```python
from build123d import *

# Parameters (mm, degrees)
SKETCH1_R           = 2.1
BOSS_EXTRUDE1_DEPTH = 1.6
SKETCH3_W           = 0.5
SKETCH3_H           = 0.75
SKETCH3_W_2         = 0.75
SKETCH3_H_2         = 0.5
CUT_EXTRUDE1_DEPTH  = 0.5
SKETCH4_R           = 1.25
BOSS_EXTRUDE2_DEPTH = 7.5


with BuildPart() as part:
    # Sketch1 → Boss-Extrude1 (new body)
    with BuildSketch(Plane.XY):
        Circle(SKETCH1_R)
    extrude(amount=BOSS_EXTRUDE1_DEPTH)

    # Sketch2 → Cut-Revolve1 (revolve, cut)
    with BuildSketch(Plane(origin=(0, 0, 0), x_dir=(1, 0, 0), z_dir=(0, 1, 0))):
        with BuildLine():
            Line((-2.1, -0.8), (-2.1, 0))
            Line((-2.1, 0), (-1.3, 0))
            ThreePointArc((-1.3, 0), (-1.865685425, -0.234314575), (-2.1, -0.8))
        make_face()
    revolve(axis=Axis((0, 0, 0), (0, 0, 1)), mode=Mode.SUBTRACT)

    # Sketch3 → Cut-Extrude1 (cut)
    with BuildSketch(Plane(origin=(0, 0, 0), x_dir=(-1, 0, 0), z_dir=(0, 0, -1))):
        with Locations((0, -0.625)):
            Rectangle(SKETCH3_W, SKETCH3_H)
        with Locations((0.625, 0)):
            Rectangle(SKETCH3_W_2, SKETCH3_H_2)
        with Locations((-0.625, 0)):
            Rectangle(SKETCH3_W_2, SKETCH3_H_2)
        with Locations((0, 0.625)):
            Rectangle(SKETCH3_W, SKETCH3_H)
        Rectangle(SKETCH3_W, SKETCH3_H_2)
    extrude(amount=-CUT_EXTRUDE1_DEPTH, mode=Mode.SUBTRACT)

    # Sketch4 → Boss-Extrude2 (add)
    with BuildSketch(Plane.XY.offset(1.6)):
        Circle(SKETCH4_R)
    extrude(amount=BOSS_EXTRUDE2_DEPTH)


solid = part.part
```
Part model, mm, in its own coordinate system. A direction names the side the tool comes from. Coordinates: 2 decimals unless noted, no trailing zeros. Order: outer loops, then holes, each group sorted by start corner. A loop starts at its lowest first (then second) coordinate and runs counter-clockwise, first axis right, second up. Notation, with made-up numbers: (39, 10) - (77, 10) arc R25 cw to (77, 39) - close; hole circle Ø1 at (52.5, 89). An arc over 180 degrees is marked (long way). Return JSON: item names as keys, results as strings. Group by question number.
Item 1: Which spindle directions (+Z, -Z, +X, -X, +Y, -Y) get a long thin tool onto all of the face, cutting with end or side? Do faces 1 (the face through (1, -1, 1.6)), 2 (the face through (2.003, 0.631, 1.194)). Say none if no direction does.
Item 2: Drill centre lines: probe 1 along X at (y, z) = (0.05, 2.25); probe 2 along Z at (x, y) = (-1, 0.9); probe 3 along Z at (x, y) = (0, -0.7). Where is each one in solid material? Low to high. Write a range as from..to.
Item 3: Cut at C-C (z = 2.5). List the corners of the cut face in (x, y).
Item 4: Pull direction X, two halves, no side cores. Call faces 3 (the face through (-0.27, -1.22, 5.3)), 4 (the face through (0, 0, 9.1)), 5 (the face through (0, 0, 0.5)): pulls with the +X half, pulls with the -X half, needs draft (parallel to the pull), parting line crosses it, or undercut.
Item 5: Cut at D-D (z = 1.25). List the corners of the cut face in (x, y), plus the area to 3 significant figures.
Item 6: Cut at A-A (y = 0). List the corners of the cut face in (x, z), plus the area to 3 significant figures.
Item 7: Pin check, flat tip, straight feed: pin 1 (1 mm diameter, centred on y = -1.5, z = 4, fed in from -X). Stop position of the tip, or through.
Check values:
{
 "1": {"face 1": "+Z", "face 2": "+Z, -Z"},
 "2": {"probe 1": "x = -1.25..1.25", "probe 2": "z = 0..1.6", "probe 3": "z = 0.5..9.1"},
 "3": {"outline": "circle Ø2.5 at (0, 0)"},
 "4": {"face 3": "parting line crosses it", "face 4": "needs draft", "face 5": "undercut"},
 "5": {"outline": "circle Ø4.2 at (0, 0)", "area": "13.9 mm2"},
 "6": {"outline": "(-2.1, 0.8) arc R0.8 ccw to (-1.3, 0) - (-1, 0) - (-1, 0.5) - (1, 0.5) - (1, 0) - (1.3, 0) arc R0.8 ccw to (2.1, 0.8) - (2.1, 1.6) - (1.25, 1.6) - (1.25, 9.1) - (-1.25, 9.1) - (-1.25, 1.6) - (-2.1, 1.6) - close", "area": "24.2 mm2"},
 "7": {"pin 1": "stops at x = -0.75"}
}
